Input: part model. Units: mm. Frame: model coordinates. A direction names the side the tool comes from. Coordinates: 2 decimals unless noted, no trailing zeros. Loops run counter-clockwise (first coordinate to the right, second up) from the corner with the lowest first, then second, coordinate; pieces in that order, holes last.
Item 1: Pull-direction query (X, two-part tool) for faces 3 (the cylindrical face through (29.577, -42.476, 2.535)), 4 (the cylindrical face through (1.5, -46.82, 2.46)), 5 (the flat face through (89, -44, 2)); classes: released by +X, released by -X, zero draft, split by the parting line, or undercut.
Item 2: Section A-A on x = 13. Return loops of the section in (y, z), and give its area (3 significant figures).
Item 3: Section C-C on x = 30.5. Return loops of the section in (y, z), and give its area (3 significant figures).
Item 4: Contact query for flat-ended pins moving along their axis: P1, Ø2.5, axis at y = -8, z = 3, coming from the +X side; P2, Ø2.5, axis at x = 97, y = 44.25, coming from the -Z side; P3, Ø0.6, axis at x = 4, y = 0.5, coming from the +Z side; P4, Ø0.9, axis at y = -45, z = 3.5, coming from the +X side. Output: stop coordinate, or through.
Item 5: Reachability of faces 1 (the cylindrical face through (8.752, 39.537, 2.465)), 2 (the cylindrical face through (100.248, 47.537, 2.465)) from +Z, -Z, +X, -X, +Y, -Y: full face, straight path, thin tool, end or side. Return the list, or none.
Item 6: Ray query, line 1 along Y through (x, z) = (70.5, 1.2); line 2 along Y through (x, z) = (12.5, 0.6); line 3 along Y through (x, z) = (97, 3.4). Return the intervals inside material, ascending.
Item 7: Section B-B on z = 1.2. Return loops of the section in (x, y).
Item 8: Section D-D on y = 20.5. Return loops of the section in (x, z).
```python
from build123d import *

# Parameters (mm, degrees)
BOSS_EXTRUDE1_DEPTH = 5
SKETCH4_R           = 2
CUT_EXTRUDE1_DEPTH  = 113.04491287
SKETCH5_R           = 1
CUT_EXTRUDE2_DEPTH  = 3


with BuildPart() as part:
    # Sketch1 → Boss-Extrude1 (new body)
    with BuildSketch(Plane.XY):
        with BuildLine():
            Line((0, -43.25), (0, 43.25))
            ThreePointArc((0, 43.25), (1.464466094, 46.785533906), (5, 48.25))
            Line((5, 48.25), (98.5, 48.25))
            ThreePointArc((98.5, 48.25), (100.267766953, 47.517766953), (101, 45.75))
            Line((101, 45.75), (101, 42.75))
            ThreePointArc((101, 42.75), (100.267766953, 40.982233047), (98.5, 40.25))
            Line((98.5, 40.25), (10.5, 40.25))
            ThreePointArc((10.5, 40.25), (8.732233047, 39.517766953), (8, 37.75))
            Line((8, 37.75), (8, -37.75))
            ThreePointArc((8, -37.75), (8.732233047, -39.517766953), (10.5, -40.25))
            Line((10.5, -40.25), (86.5, -40.25))
            ThreePointArc((86.5, -40.25), (88.267766953, -40.982233047), (89, -42.75))
            Line((89, -42.75), (89, -45.75))
            ThreePointArc((89, -45.75), (88.267766953, -47.517766953), (86.5, -48.25))
            Line((86.5, -48.25), (5, -48.25))
            ThreePointArc((5, -48.25), (1.464466094, -46.785533906), (0, -43.25))
        make_face()
    extrude(amount=BOSS_EXTRUDE1_DEPTH)

    # Sketch4 → Cut-Extrude1 (cut, through all)
    with BuildSketch(Plane.XY.offset(5)):
        with Locations((70.5, 44.25)):
            Circle(SKETCH4_R)
        with Locations((30.5, 44.25)):
            Circle(SKETCH4_R)
        with Locations(Location((70.5, -44.25, 0), (0, 0, 180))):
            Circle(SKETCH4_R)
        with Locations(Location((30.5, -44.25, 0), (0, 0, 180))):
            Circle(SKETCH4_R)
        with Locations((50.5, 44.25)):
            Circle(SKETCH4_R)
    extrude(amount=-CUT_EXTRUDE1_DEPTH, mode=Mode.SUBTRACT)

    # Sketch5 → Cut-Extrude2 (cut)
    with BuildSketch(Plane.XY.offset(5)):
        with Locations((4, 44.25)):
            Circle(SKETCH5_R)
        with Locations((4, 0)):
            Circle(SKETCH5_R)
        with Locations((4, -44.25)):
            Circle(SKETCH5_R)
        with Locations((97, 44.25)):
            Circle(SKETCH5_R)
    extrude(amount=-CUT_EXTRUDE2_DEPTH, mode=Mode.SUBTRACT)


solid = part.part
```
Results found:
1. face 3: undercut
1. face 4: released by -X
1. face 5: released by +X
2. outline: (-48.25, 0) - (-40.25, 0) - (-40.25, 5) - (-48.25, 5) - close; (40.25, 0) - (48.25, 0) - (48.25, 5) - (40.25, 5) - close
2. area: 80.0 mm2
3. outline: (-48.25, 0) - (-46.25, 0) - (-46.25, 5) - (-48.25, 5) - close; (-42.25, 0) - (-40.25, 0) - (-40.25, 5) - (-42.25, 5) - close; (40.25, 0) - (42.25, 0) - (42.25, 5) - (40.25, 5) - close; (46.25, 0) - (48.25, 0) - (48.25, 5) - (46.25, 5) - close
3. area: 40.0 mm2
4. P1: stops at x = 8
4. P2: stops at z = 0
4. P3: stops at z = 2
4. P4: stops at x = 89
5. face 1: +Z, -Z, +X
5. face 2: +Z, -Z, +X, +Y
6. line 1: y = -48.25 to -46.25, -42.25 to -40.25, 40.25 to 42.25, 46.25 to 48.25
6. line 2: y = -48.25 to -40.25, 40.25 to 48.25
6. line 3: y = 40.25 to 43.25, 45.25 to 48.25
7. outline: (0, -43.25) arc R5 ccw to (5, -48.25) - (86.5, -48.25) arc R2.5 ccw to (89, -45.75) - (89, -42.75) arc R2.5 ccw to (86.5, -40.25) - (10.5, -40.25) arc R2.5 cw to (8, -37.75) - (8, 37.75) arc R2.5 cw to (10.5, 40.25) - (98.5, 40.25) arc R2.5 ccw to (101, 42.75) - (101, 45.75) arc R2.5 ccw to (98.5, 48.25) - (5, 48.25) arc R5 ccw to (0, 43.25) - close; hole circle Ø4 at (30.5, -44.25); hole circle Ø4 at (30.5, 44.25); hole circle Ø4 at (50.5, 44.25); hole circle Ø4 at (70.5, -44.25); hole circle Ø4 at (70.5, 44.25)
8. outline: (0, 0) - (8, 0) - (8, 5) - (0, 5) - close
